```python
from build123d import *

# Parameters (mm, degrees)
SKETCH1_W               = 20
SKETCH1_H               = 20
BOSS_EXTRUDE1_DEPTH     = 77.5
SKETCH2_W               = 20
SKETCH2_H               = 20
BOSS_EXTRUDE2_DEPTH     = 2.5
CUT_EXTRUDE1_DEPTH      = 78.569323834
CUT_EXTRUDE1_DEPTH_BACK = 78.569323834
SKETCH3_R               = 1.5
CHAMFER1_SIZE           = 1.5
CHAMFER2_SIZE           = 1
FILLET1_R               = 1.5


with BuildPart() as part:
    # Sketch1 → Boss-Extrude1 (new body)
    with BuildSketch(Plane(origin=(0, 0, 0), x_dir=(1, 0, 0), z_dir=(0, 1, 0))):
        Polygon((-11, 2.116025404), (-11, -2.116025404), (-12.5, -1.25), (-12.5, -12.5), (-1, -12.5), (-1.866025404, -14), (1.866025404, -14), (1, -12.5), (12.5, -12.5), (12.5, -1), (14, -1.866025404), (14, 1.866025404), (12.5, 1), (12.5, 12.5), (1.25, 12.5), (2.116025404, 11), (-2.116025404, 11), (-1.25, 12.5), (-12.5, 12.5), (-12.5, 1.25), align=None)
        Rectangle(SKETCH1_W, SKETCH1_H, mode=Mode.SUBTRACT)
    extrude(amount=BOSS_EXTRUDE1_DEPTH)

    # Sketch2 → Boss-Extrude2 (add)
    with BuildSketch(Plane(origin=(0, 0, 0), x_dir=(1, 0, 0), z_dir=(0, 1, 0))):
        Rectangle(SKETCH2_W, SKETCH2_H)
    extrude(amount=BOSS_EXTRUDE2_DEPTH)

    # Sketch3 → Cut-Extrude1 (cut, two sides: drawn at the far end of the back side and taken through both)
    with BuildSketch(Plane(origin=(0, 2.5, 0), x_dir=(1, 0, 0), z_dir=(0, 1, 0)).offset(-CUT_EXTRUDE1_DEPTH_BACK)):
        with Locations(Location((-6, 6, 0), (0, 0, 270))):
            Circle(SKETCH3_R)
        with Locations(Location((6, 6, 0), (0, 0, 90))):
            Circle(SKETCH3_R)
        with Locations(Location((6, -6, 0), (0, 0, 270))):
            Circle(SKETCH3_R)
        with Locations(Location((-6, -6, 0), (0, 0, 90))):
            Circle(SKETCH3_R)
    extrude(amount=CUT_EXTRUDE1_DEPTH + CUT_EXTRUDE1_DEPTH_BACK, mode=Mode.SUBTRACT)

    # Chamfer1
    chamfer1_edges = [part.edges().sort_by_distance(p)[0] for p in [
        (14, 0, 0),
        (12.5, 0, -6.75),
        (6.875, 0, -12.5),
        (0, 0, -11),
        (0, 0, 14),
        (12.5, 0, 6.75),
        (6.75, 0, 12.5),
        (-11, 0, 0),
        (-6.75, 0, 12.5),
        (-12.5, 0, 6.875),
        (-6.875, 0, -12.5),
        (-12.5, 0, -6.875),
    ]]
    chamfer(chamfer1_edges, length=CHAMFER1_SIZE - 0.0001)  # a hair under: the kernel refuses the full size

    # Chamfer2
    chamfer2_edges = [part.edges().sort_by_distance(p)[0] for p in [
        (0, 2.5, -10),
        (-10, 2.5, 0),
        (0, 2.5, 10),
        (10, 2.5, 0),
        (-6, 2.5, 7.5),
        (6, 2.5, 4.5),
        (6, 2.5, -4.5),
        (-6, 2.5, -7.5),
    ]]
    chamfer(chamfer2_edges, length=CHAMFER2_SIZE)

    # Fillet1
    fillet1_edges = [part.edges().sort_by_distance(p)[0] for p in [
        (10, 40.5, -10),
        (-10, 40.5, -10),
        (-10, 40.5, 10),
        (10, 40.5, 10),
    ]]
    fillet(fillet1_edges, radius=FILLET1_R)


solid = part.part
```
The listing builds one solid part. Answer for the finished solid, in the listing's coordinates (mm). A direction names the side the tool comes from. Round coordinates to 2 decimals unless told otherwise and drop trailing zeros. Order: outer loops, then holes, each group sorted by start corner. A loop starts at its lowest first (then second) coordinate and runs counter-clockwise, first axis right, second up. Notation, with made-up numbers: (42.5, 82) - (51.5, 82) arc R17 cw to (51.5, 110) - close; hole circle Ø7 at (84.25, -23.5). An arc over 180 degrees is marked (long way). Put each result on its own line as item: value. Start each with the question number.
(1) Determine the mould class of faces 4 (the flat face through (-11.688, 38.207, -1.719)), 5 (the flat face through (-7, 1, -12)), 6 (the flat face through (-12.5, 39, -7)) for opening direction X: released by +X, released by -X, zero draft, split by the parting line, or undercut.
(2) For faces 1 (the cylindrical face through (-9.55, 40.8, -9.57)), 2 (the flat face through (-11, 39, 0)), 3 (the flat face through (13.3, 0.8, 0)), determine the directions among +Z, -Z, +X, -X, +Y, -Y from which every point of the face is accessible in a straight line to the end or side of a thin tool.
(3) Find section C-C (z = -6). Give the vertices of the cut face in (x, y), plus the area to 3 significant figures.
(4) Given P1, Ø5, axis at x = -7, y = 19.5, coming from the +Z side; P2, Ø9, axis at y = 47, z = 6.5, coming from the +X side; P3, Ø3.5, axis at x = -6, z = 6, coming from the +Y side, each flat-ended and moving along its own axis, determine where each tip first touches the part or whether it passes through.
(5) Find section B-B (y = 73). Give the vertices of the cut face in (x, z).
(6) Straight lines are drawn through the part: probe 1 along X at (y, z) = (44, -8.25); probe 2 along Z at (x, y) = (0, 74.5). For each, find the intervals that lie inside material, in ascending order. Write a range as from..to.
(7) Find section A-A (x = -6). Give the vertices of the cut face in (y, z).
Reply:
1. face 4: undercut
1. face 5: zero draft
1. face 6: released by -X
2. face 1: +Y
2. face 2: +Y, -Y
2. face 3: +Z, -Z, +X, -Y
3. outline: (-12.5, 1.5) - (-11, 0) - (-7.5, 0) - (-7.5, 1.5) - (-8.5, 2.5) - (-9, 2.5) - (-10, 3.5) - (-10, 77.5) - (-12.5, 77.5) - close; (-4.5, 0) - (4.5, 0) - (4.5, 1.5) - (3.5, 2.5) - (-3.5, 2.5) - (-4.5, 1.5) - close; (7.5, 0) - (11, 0) - (12.5, 1.5) - (12.5, 77.5) - (10, 77.5) - (10, 3.5) - (9, 2.5) - (8.5, 2.5) - (7.5, 1.5) - close
3. area: 419 mm^2
4. P1: z = 12.5
4. P2: x = 12.5
4. P3: y = 1.75
5. outline: (-12.5, -12.5) - (-1.25, -12.5) - (-2.12, -11) - (2.12, -11) - (1.25, -12.5) - (12.5, -12.5) - (12.5, -1) - (14, -1.87) - (14, 1.87) - (12.5, 1) - (12.5, 12.5) - (1, 12.5) - (1.87, 14) - (-1.87, 14) - (-1, 12.5) - (-12.5, 12.5) - (-12.5, 1.25) - (-11, 2.12) - (-11, -2.12) - (-12.5, -1.25) - close; hole (-10, -8.5) arc R1.5 ccw to (-8.5, -10) - (8.5, -10) arc R1.5 ccw to (10, -8.5) - (10, 8.5) arc R1.5 ccw to (8.5, 10) - (-8.5, 10) arc R1.5 ccw to (-10, 8.5) - close
6. probe 1: -12.5..-10, 10..12.5
6. probe 2: -11..-10, 10..14
7. outline: (0, -11) - (1.5, -12.5) - (77.5, -12.5) - (77.5, -10) - (3.5, -10) - (2.5, -9) - (2.5, -8.5) - (1.5, -7.5) - (0, -7.5) - close; (0, -4.5) - (1.5, -4.5) - (2.5, -3.5) - (2.5, 3.5) - (1.5, 4.5) - (0, 4.5) - close; (0, 7.5) - (1.5, 7.5) - (2.5, 8.5) - (2.5, 9) - (3.5, 10) - (77.5, 10) - (77.5, 12.5) - (1.5, 12.5) - (0, 11) - close
